CAD build for the part. Positions are in the model's coordinates, mm. Face numbers are marked on the shaded views. Coordinates: 2 decimals unless noted, no trailing zeros. Order: outer loops, then holes, each group sorted by start corner. A loop starts at its lowest first (then second) coordinate and runs counter-clockwise, first axis right, second up. Notation, with made-up numbers: M 73.25,67 L 130.25,67 A25 cw 130.25,99 Z; hole C 35.25,72.25 d9. An arc over 180 degrees is marked long. Write item = value, one per line.
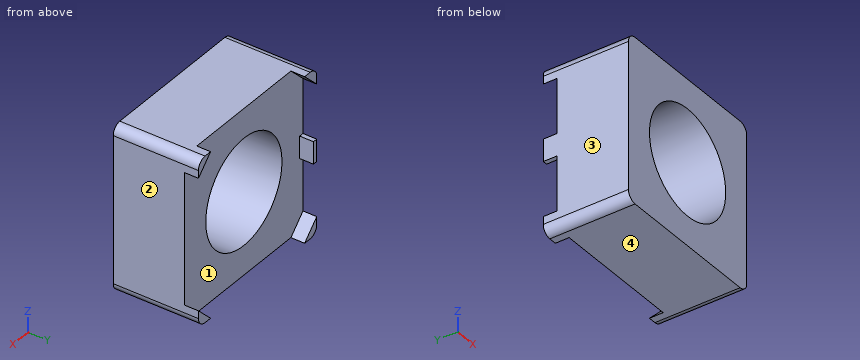
Autodesk Inventor part; units mm, degrees
ref_plane "YZ Plane" through (0, 0, 0) normal (1, 0, 0) x (0, 1, 0)
ref_plane "XZ Plane" through (0, 0, 0) normal (0, 1, 0) x (-1, 0, 0)
ref_plane "XY Plane" through (0, 0, 0) normal (0, 0, 1) x (1, 0, 0)
sketch "Skizze1" plane through (0, 0, 0) normal (0, 1, 0) x (-1, 0, 0)
  line L0 (-9, -9) -> (9, -9)
  line L1 (9, -9) -> (9, 9)
  line L2 (9, 9) -> (-9, 9)
  line L3 (-9, 9) -> (-9, -9)
  line L4 (-9, -9) -> (9, 9) construction
  line L5 (9, -9) -> (-9, 9) construction
  circle A0 centre (0, 0) radius 5.8
  dimension "d0" = 18
  dimension "d1" = 18
  dimension "d2" = 11.6
extrude "Extrusion1" add sketch "Skizze1" along normal blind 7.8
sketch "Skizze2" plane through (0, 7.8, 0) normal (0, 1, 0) x (1, 0, 0)
  line L0 (-9, 9) -> (-9, -9)
  line L1 (-9, -9) -> (9, -9)
  line L2 (9, -9) -> (9, 9)
  line L3 (9, 9) -> (-9, 9)
  circle A0 centre (0, 0) radius 5.8
  line L4 (-9, 9) -> (-9, -9)
  line L5 (-9, -7.1615) -> (-7.1615, -9)
  line L6 (-9, -7.1615) -> (-6.4, -7.1615) construction
  dimension "d5" = 45
  dimension "d6" = 1.3
extrude "Extrusion2" add sketch "Skizze2" along normal blind 1.5 contours L5 L1 L0
pattern_circular "Runde Anordnung1" count 4 over 360 about axis through (0, 0, 0) along (0, 1, 0) of "Extrusion2"
fillet "Rundung1" radius 1 4 edges at (-9, 4.65, 9) (9, 4.65, 9) (9, 4.65, -9) (-9, 4.65, -9)
sketch "Skizze3" plane through (-9, 7.8, 7.1615) normal (-1, 0, 0) x (0, 0, 1)
  line L0 (-15.1615, -7.8) -> (-15.1615, 1.5)
  line L1 (-15.1615, -7.8) -> (0.8385, -7.8)
  line L2 (0.8385, 1.5) -> (0.8385, -7.8)
  line L3 (0, 1.5) -> (0.8385, 1.5)
  line L4 (0, 0) -> (0, 1.5)
  line L5 (-14.323, 0) -> (0, 0)
  line L6 (-14.323, 0) -> (-14.323, 1.5)
  line L7 (-15.1615, 1.5) -> (-14.323, 1.5)
  line L8 (-8.3736, -1.5) -> (-5.9495, -1.5)
  line L9 (-5.9495, -1.5) -> (-5.9495, 1.5)
  line L10 (-5.9495, 1.5) -> (-8.3736, 1.5)
  line L11 (-8.3736, 1.5) -> (-8.3736, -1.5)
  line L12 (-14.323, 0) -> (0, 0)
  line L13 (-8.3736, -1.5) -> (-5.9495, 1.5) construction
  line L14 (-5.9495, -1.5) -> (-8.3736, 1.5) construction
  point P0 (-7.1615, -7.8)
  point P1 (-7.1615, 0)
extrude "Extrusion3" add sketch "Skizze3" against normal blind 0.5 contours L11 L10 L9 L5 | L5 L9 L8 L11
properties part number "00_VCM_M12"
(1) Slice it at A-A, the plane z = 0. Write the cut outline in (x, y).
Evaluation:
outline = M -9,0 L -5.8,0 L -5.8,7.8 L -8.5,7.8 L -8.5,9.3 L -9,9.3 Z; M 5.8,0 L 9,0 L 9,7.8 L 5.8,7.8 Z
(2) Slice it at C-C, the plane y = 7.5. Write the cut outline in (x, z).
Evaluation:
outline = M -9,-8 A1 ccw -8,-9 L 8,-9 A1 ccw 9,-8 L 9,8 A1 ccw 8,9 L -8,9 A1 ccw -9,8 Z; hole C 0,0 d11.6
(3) Slice it at D-D, the plane x = -7.5. Write the cut outline in (y, z), then the cut area to 3 significant figures.
Evaluation:
outline = M 0,-9 L 9.3,-9 L 9.3,-8.66 L 7.8,-8.66 L 7.8,8.66 L 9.3,8.66 L 9.3,9 L 0,9 Z
area = 141 mm²
(4) Slice it at B-B, the plane x = 0. Write the cut outline in (y, z), then the cut area to 3 significant figures.
Evaluation:
outline = M 0,-9 L 7.8,-9 L 7.8,-5.8 L 0,-5.8 Z; M 0,5.8 L 7.8,5.8 L 7.8,9 L 0,9 Z
area = 49.9 mm²
(5) Pin check, flat tips, straight feed: pin 1 Ø1 at (x, z) = (5.5, 5) entering from +Y; pin 2 Ø1.7 at (y, z) = (8.5, 0.5) entering from +X. Stop position of each tip, or through.
Evaluation:
pin_1 = 7.8
pin_2 = 9
(6) Pull direction X, two halves, no side cores. Call the marked faces 1, 2, 3 and 4: +X half, -X half, draft (parallel to the pull), parting line (faces both ways), or undercut.
Evaluation:
face_1 = undercut
face_2 = +X half
face_3 = -X half
face_4 = draft
(7) Wall check: line 1 (Z direction, x = 0, y = 4); line 2 (Y direction, x = -8, z = 3); line 3 (X direction, y = 8.25, z = -8). Give the ranges that are in metal, low to high. Write a range as from..to.
Evaluation:
line_1 = -9..-5.8, 5.8..9
line_2 = 0..7.8
line_3 = -9..-8.16, 8.16..9
